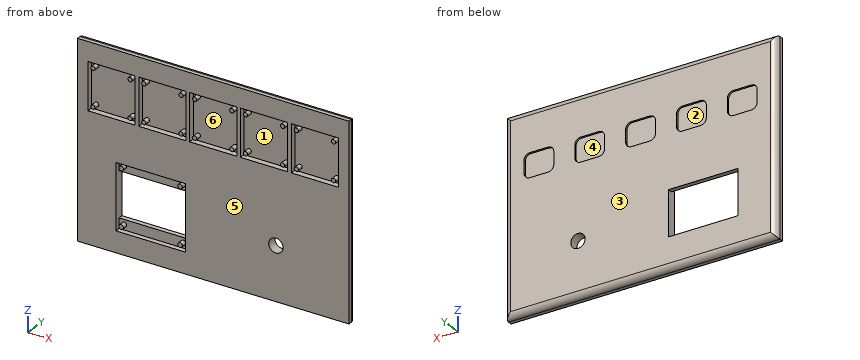
```python
from build123d import *

# Parameters (mm, degrees)
SKETCH1_W           = 140.4
SKETCH1_H           = 100.4
SKETCH1_W_2         = 35.9
SKETCH1_H_2         = 33.9
SKETCH1_R           = 3.7
BOSS_EXTRUDE1_DEPTH = 5
FILLET1_R           = 3
SKETCH3_W           = 35.9
SKETCH3_H           = 5.25
BOSS_EXTRUDE2_DEPTH = 2.4
BOSS_EXTRUDE3_START = -2.6
SKETCH4_R           = 1.2
BOSS_EXTRUDE3_DEPTH = 2.6
SKETCH6_W           = 24.4
SKETCH6_H           = 24.4
CUT_EXTRUDE1_DEPTH  = 3
LPATTERN1_COUNT     = 5
LPATTERN1_PITCH     = 26.3
SKETCH7_R           = 1.1
BOSS_EXTRUDE4_DEPTH = 3
LPATTERN2_COUNT     = 5
LPATTERN2_PITCH     = 26.3
SKETCH9_W           = 15.4
SKETCH9_H           = 12.4
BOSS_EXTRUDE5_DEPTH = 1
LPATTERN3_COUNT     = 5
LPATTERN3_PITCH     = 26.3


with BuildPart() as part:
    # Sketch1 → Boss-Extrude1 (new body)
    with BuildSketch(Plane(origin=(0, 0, 0), x_dir=(1, 0, 0), z_dir=(0, 1, 0))):
        with Locations((0.704074767, -0.111023374)):
            Rectangle(SKETCH1_W, SKETCH1_H)
        with Locations((-31.695925233, 22.288976626)):
            Rectangle(SKETCH1_W_2, SKETCH1_H_2, mode=Mode.SUBTRACT)
        with Locations(Location((33.104074767, 22.288976626, 0), (0, 0, 270))):
            Circle(SKETCH1_R, mode=Mode.SUBTRACT)
        with BuildLine():
            Line((-47.195925233, -28.711023374), (-56.595925233, -28.711023374))
            ThreePointArc((-56.595925233, -28.711023374), (-58.717245577, -27.832343717), (-59.595925233, -25.711023374))
            Line((-59.595925233, -25.711023374), (-59.595925233, -19.311023374))
            ThreePointArc((-59.595925233, -19.311023374), (-58.717245577, -17.18970303), (-56.595925233, -16.311023374))
            Line((-56.595925233, -16.311023374), (-47.195925233, -16.311023374))
            ThreePointArc((-47.195925233, -16.311023374), (-45.07460489, -17.18970303), (-44.195925233, -19.311023374))
            Line((-44.195925233, -19.311023374), (-44.195925233, -25.711023374))
            ThreePointArc((-44.195925233, -25.711023374), (-45.07460489, -27.832343717), (-47.195925233, -28.711023374))
        make_face(mode=Mode.SUBTRACT)
        with BuildLine():
            ThreePointArc((-33.295925233, -19.311023374), (-32.417245577, -17.18970303), (-30.295925233, -16.311023374))
            Line((-30.295925233, -16.311023374), (-20.895925233, -16.311023374))
            ThreePointArc((-20.895925233, -16.311023374), (-18.77460489, -17.18970303), (-17.895925233, -19.311023374))
            Line((-17.895925233, -19.311023374), (-17.895925233, -25.711023374))
            ThreePointArc((-17.895925233, -25.711023374), (-18.77460489, -27.832343717), (-20.895925233, -28.711023374))
            Line((-20.895925233, -28.711023374), (-30.295925233, -28.711023374))
            ThreePointArc((-30.295925233, -28.711023374), (-32.417245577, -27.832343717), (-33.295925233, -25.711023374))
            Line((-33.295925233, -25.711023374), (-33.295925233, -19.311023374))
        make_face(mode=Mode.SUBTRACT)
        with BuildLine():
            ThreePointArc((-6.995925233, -19.311023374), (-6.117245577, -17.18970303), (-3.995925233, -16.311023374))
            Line((-3.995925233, -16.311023374), (5.404074767, -16.311023374))
            ThreePointArc((5.404074767, -16.311023374), (7.52539511, -17.18970303), (8.404074767, -19.311023374))
            Line((8.404074767, -19.311023374), (8.404074767, -25.711023374))
            ThreePointArc((8.404074767, -25.711023374), (7.52539511, -27.832343717), (5.404074767, -28.711023374))
            Line((5.404074767, -28.711023374), (-3.995925233, -28.711023374))
            ThreePointArc((-3.995925233, -28.711023374), (-6.117245577, -27.832343717), (-6.995925233, -25.711023374))
            Line((-6.995925233, -25.711023374), (-6.995925233, -19.311023374))
        make_face(mode=Mode.SUBTRACT)
        with BuildLine():
            ThreePointArc((19.304074767, -19.311023374), (20.182754423, -17.18970303), (22.304074767, -16.311023374))
            Line((22.304074767, -16.311023374), (31.704074767, -16.311023374))
            ThreePointArc((31.704074767, -16.311023374), (33.82539511, -17.18970303), (34.704074767, -19.311023374))
            Line((34.704074767, -19.311023374), (34.704074767, -25.711023374))
            ThreePointArc((34.704074767, -25.711023374), (33.82539511, -27.832343717), (31.704074767, -28.711023374))
            Line((31.704074767, -28.711023374), (22.304074767, -28.711023374))
            ThreePointArc((22.304074767, -28.711023374), (20.182754423, -27.832343717), (19.304074767, -25.711023374))
            Line((19.304074767, -25.711023374), (19.304074767, -19.311023374))
        make_face(mode=Mode.SUBTRACT)
        with BuildLine():
            ThreePointArc((45.604074767, -19.311023374), (46.482754423, -17.18970303), (48.604074767, -16.311023374))
            Line((48.604074767, -16.311023374), (58.004074767, -16.311023374))
            ThreePointArc((58.004074767, -16.311023374), (60.12539511, -17.18970303), (61.004074767, -19.311023374))
            Line((61.004074767, -19.311023374), (61.004074767, -25.711023374))
            ThreePointArc((61.004074767, -25.711023374), (60.12539511, -27.832343717), (58.004074767, -28.711023374))
            Line((58.004074767, -28.711023374), (48.604074767, -28.711023374))
            ThreePointArc((48.604074767, -28.711023374), (46.482754423, -27.832343717), (45.604074767, -25.711023374))
            Line((45.604074767, -25.711023374), (45.604074767, -19.311023374))
        make_face(mode=Mode.SUBTRACT)
    extrude(amount=BOSS_EXTRUDE1_DEPTH)

    # Fillet1
    fillet1_edges = [part.edges().sort_by_distance(p)[0] for p in [
        (0.704074767, 5, 50.311023374),
        (70.904074767, 5, 0.111023374),
        (0.704074767, 5, -50.088976626),
        (-69.495925233, 5, 0.111023374),
    ]]
    fillet(fillet1_edges, radius=FILLET1_R)

    # Sketch3 → Boss-Extrude2 (add)
    with BuildSketch(Plane(origin=(0, 5, 0), x_dir=(1, 0, 0), z_dir=(0, 1, 0))):
        with Locations((-31.695925233, 36.613976626)):
            Rectangle(SKETCH3_W, SKETCH3_H)
        with Locations((-31.695925233, 7.963976626)):
            Rectangle(SKETCH3_W, SKETCH3_H)
    extrude(amount=-BOSS_EXTRUDE2_DEPTH)

    # Sketch4 → Boss-Extrude3 (add)
    with BuildSketch(Plane.XZ.offset(BOSS_EXTRUDE3_START)):
        with Locations(Location((-16.445925233, -36.538976626, 0), (0, 0, 90))):
            Circle(SKETCH4_R)
        with Locations(Location((-46.945925233, -36.538976626, 0), (0, 0, 90))):
            Circle(SKETCH4_R)
        with Locations(Location((-16.445925233, -7.538976626, 0), (0, 0, 90))):
            Circle(SKETCH4_R)
        with Locations(Location((-46.945925233, -7.538976626, 0), (0, 0, 90))):
            Circle(SKETCH4_R)
    extrude(amount=BOSS_EXTRUDE3_DEPTH)

    # Sketch6 → Cut-Extrude1 (cut)
    with BuildSketch(Plane.XZ):
        with Locations((-51.895925233, 28.211023374)):
            Rectangle(SKETCH6_W, SKETCH6_H)
    cut_extrude1 = extrude(amount=-CUT_EXTRUDE1_DEPTH, mode=Mode.SUBTRACT)

    # LPattern1: Cut-Extrude1 ×5
    with Locations(*[(i * LPATTERN1_PITCH, 0, 0) for i in range(1, LPATTERN1_COUNT)]):
        add(cut_extrude1, mode=Mode.SUBTRACT)

    # Sketch7 → Boss-Extrude4 (add)
    with BuildSketch(Plane.XZ.offset(-3)):
        with Locations(Location((-61.495925233, 37.811023374, 0), (0, 0, 90))):
            Circle(SKETCH7_R)
        with Locations(Location((-42.295925233, 37.811023374, 0), (0, 0, 90))):
            Circle(SKETCH7_R)
        with Locations(Location((-61.495925233, 18.611023374, 0), (0, 0, 90))):
            Circle(SKETCH7_R)
        with Locations(Location((-42.295925233, 18.611023374, 0), (0, 0, 90))):
            Circle(SKETCH7_R)
    boss_extrude4 = extrude(amount=BOSS_EXTRUDE4_DEPTH)

    # LPattern2: Boss-Extrude4 ×5
    with Locations(*[(i * LPATTERN2_PITCH, 0, 0) for i in range(1, LPATTERN2_COUNT)]):
        add(boss_extrude4)

    # Sketch9 → Boss-Extrude5 (add)
    with BuildSketch(Plane.XZ.offset(-3)):
        with Locations((-51.895925233, 22.511023374)):
            Rectangle(SKETCH9_W, SKETCH9_H)
    boss_extrude5 = extrude(amount=-BOSS_EXTRUDE5_DEPTH)

    # LPattern3: Boss-Extrude5 ×5
    with Locations(*[(i * LPATTERN3_PITCH, 0, 0) for i in range(1, LPATTERN3_COUNT)]):
        add(boss_extrude5)


solid = part.part
```
Check sheet for the modelled part. Datum: model origin and axes. Units: mm. Face numbers are marked on the shaded views. A direction names the side the tool comes from. Round coordinates to 2 decimals unless told otherwise and drop trailing zeros. Order: outer loops, then holes, each group sorted by start corner. A loop starts at its lowest first (then second) coordinate and runs counter-clockwise, first axis right, second up. Notation, with made-up numbers: (81, -24) - (96, -24) arc R23 ccw to (96, 14) - close; hole circle Ø4 at (85, 56.5). An arc over 180 degrees is marked (long way). Write item = value, one per line.
Q1. Go/stop test with flat-tipped pins: pin 1 (1.2 mm diameter, centred on x = -36, y = 3, fed in from +Z); pin 2 (7.5 mm diameter, centred on x = -53, z = 28, fed in from -Y); pin 3 (0.8 mm diameter, centred on x = 52.5, y = 4.5, fed in from -Z). Record where each tip stops, or that it passes through.
Computed:
pin_1 = 50.28
pin_2 = 3
pin_3 = -49.23
Q2. Tool access check on the marked faces 1, 2 and 3. Record the directions out of +Z, -Z, +X, -X, +Y, -Y that give a thin tool (end or side, any length) a straight path to the whole face; none if there is none.
Computed:
face_1 = -Y
face_2 = +Y
face_3 = +Z, -Z, +X, -X, +Y
Q3. Thickness scan on line 1 along X through (y, z) = (0.8, -14.5); line 2 along Z through (x, y) = (33.5, 1.25); line 3 along Z through (x, y) = (56, 2.1). Record the ranges inside material, lowest first.
Computed:
line_1 = -69.5 to -49.65, -13.75 to 70.9
line_2 = -50.09 to -25.97, -18.61 to 16.01, 40.41 to 50.31
line_3 = -50.09 to 16.01, 40.41 to 50.31
Q4. Section check A-A (z = -32). Record the boundary of the cut face in (x, y).
Computed:
outline = (-69.5, 0) - (-49.65, 0) - (-49.65, 5) - (-66.5, 5) arc R3 ccw to (-69.5, 2) - close; (-13.75, 0) - (70.9, 0) - (70.9, 2) arc R3 ccw to (67.9, 5) - (-13.75, 5) - close
Q5. Draft check along Z on the marked faces 4, 5 and 6. Enter one of: pulls with the +Z half, pulls with the -Z half, needs draft (parallel to the pull), parting line crosses it, or undercut.
Computed:
face_4 = undercut
face_5 = needs draft
face_6 = undercut
